```python
from build123d import *

# Parameters (mm, degrees)
SKETCH1_R           = 10
BOSS_EXTRUDE1_DEPTH = 105
BOSS_EXTRUDE2_DEPTH = 15


with BuildPart() as part:
    # Sketch1 → Boss-Extrude1 (new body)
    with BuildSketch(Plane(origin=(0, 0, 0), x_dir=(1, 0, 0), z_dir=(0, 1, 0))):
        Circle(SKETCH1_R)
    extrude(amount=BOSS_EXTRUDE1_DEPTH)

    # Sketch2 → Boss-Extrude2 (add)
    with BuildSketch(Plane(origin=(0, 105, 0), x_dir=(1, 0, 0), z_dir=(0, 1, 0))):
        Polygon((20.207259422, 0), (10.103629711, 17.5), (-10.103629711, 17.5), (-20.207259422, 0), (-10.103629711, -17.5), (10.103629711, -17.5), align=None)
    extrude(amount=-BOSS_EXTRUDE2_DEPTH)

    # Sketch3 → Cut-Revolve1 (revolve, cut)
    with BuildSketch(Plane.XY):
        Polygon((20.207259422, 105), (20.207259422, 102), (17.207259422, 105), align=None)
    revolve(axis=Axis((0, 0, 0), (0, 1, 0)), mode=Mode.SUBTRACT)


solid = part.part
```
For this review, take the finished solid that the model builds, in its own axes (mm). A direction names the side the tool comes from. Coordinates: 2 decimals unless noted, no trailing zeros. Write each loop counter-clockwise with the first axis right and the second up, starting at its lowest first coordinate (ties: lowest second). Pieces come first, ordered by that corner, then holes.
(1) Tool access review of faces 1 (the face through (-2.17, 44.37, 9.76)), 2 (the face through (0, 0, 0)): name each direction out of +Z, -Z, +X, -X, +Y, -Y from which nothing blocks a thin tool from reaching the whole face with its end or side.
(2) For pin 1 Ø8 at (y, z) = (12.5, -10.5) entering from +X; pin 2 Ø3 at (y, z) = (31.5, -6.5) entering from -X; pin 3 Ø5 at (x, y) = (1, 72) entering from +Z, all flat-tipped, find the tip position at first contact; note any pin that passes through.
(3) Add section B-B on y = 33. Give the boundary of the cut face in (x, z), then the cut area to 3 significant figures.
(4) Wall thickness on probe 1 along Y at (x, z) = (10, -3.5); probe 2 along Z at (x, y) = (0, 38); probe 3 along Y at (x, z) = (12, -12.5): over which ranges is each line inside the solid? List them lowest first.
(5) Add section A-A on x = 0. Give the boundary of the cut face in (y, z).
Answer sheet:
1. face 1: -Y
1. face 2: +Z, -Z, +X, -X, -Y
2. pin 1: stops at x = 7.6
2. pin 2: stops at x = -8.66
2. pin 3: stops at z = 10
3. outline: circle Ø20 at (0, 0)
3. area: 314 mm2
4. probe 1: y = 90 to 105
4. probe 2: z = -10 to 10
4. probe 3: y = 90 to 104.88
5. outline: (0, -10) - (90, -10) - (90, -17.5) - (104.71, -17.5) - (105, -17.21) - (105, 17.21) - (104.71, 17.5) - (90, 17.5) - (90, 10) - (0, 10) - close
